Geometry: final body of the model. Coordinates: model frame, mm. Give positions to 0.01 mm unless a question says otherwise; leave off trailing zeros. Order: outer loops, then holes, each group sorted by start corner. A loop starts at its lowest first (then second) coordinate and runs counter-clockwise, first axis right, second up. Notation, with made-up numbers: (10, 19) -> (27, 19) arc R32 ccw to (27, 52) -> close; hole circle Ø6 at (63, 2). An arc over 180 degrees is marked (long way). Write item = value, one per line.
```python
from build123d import *

# Parameters (mm, degrees)
SKETCH1_R           = 1.8
BOSS_EXTRUDE1_DEPTH = 3


with BuildPart() as part:
    # Sketch1 → Boss-Extrude1 (new body)
    with BuildSketch(Plane(origin=(0, 0, 0), x_dir=(1, 0, 0), z_dir=(0, 1, 0))):
        with BuildLine():
            Line((11, 44), (11, 70))
            Line((11, 70), (0, 70))
            Line((0, 70), (0, 0))
            Line((0, 0), (11, 0))
            Line((11, 0), (11, 26))
            ThreePointArc((11, 26), (6.32455532, 35), (11, 44))
        make_face()
        with Locations((5.5, 65.5)):
            Circle(SKETCH1_R, mode=Mode.SUBTRACT)
        with Locations((5.5, 4.5)):
            Circle(SKETCH1_R, mode=Mode.SUBTRACT)
        with Locations((5.5, 19.5)):
            Circle(SKETCH1_R, mode=Mode.SUBTRACT)
        with Locations((5.5, 50.5)):
            Circle(SKETCH1_R, mode=Mode.SUBTRACT)
    extrude(amount=BOSS_EXTRUDE1_DEPTH)


solid = part.part
```
1) Section query A-A (x = 5.5). Output: boundary loops of the cut face in (y, z).
Check sheet entries:
outline = (0, -70) -> (3, -70) -> (3, -67.3) -> (0, -67.3) -> close; (0, -63.7) -> (3, -63.7) -> (3, -52.3) -> (0, -52.3) -> close; (0, -48.7) -> (3, -48.7) -> (3, -21.3) -> (0, -21.3) -> close; (0, -17.7) -> (3, -17.7) -> (3, -6.3) -> (0, -6.3) -> close; (0, -2.7) -> (3, -2.7) -> (3, 0) -> (0, 0) -> close
2) Mould query, pull axis Z, two halves, no side actions, for faces 1 (the face through (5.266, 1.479, -52.285)), 2 (the face through (11, 1, -57)), 3 (the face through (5, 1, 0)). Classes: +Z half, -Z half, draft (parallel to the pull), parting line (faces both ways), or undercut.
Check sheet entries:
face_1 = undercut
face_2 = draft
face_3 = +Z half
3) Section query B-B (z = -65.5). Output: boundary loops of the cut face in (x, y), plus the area to 3 significant figures.
Check sheet entries:
outline = (0, 0) -> (3.7, 0) -> (3.7, 3) -> (0, 3) -> close; (7.3, 0) -> (11, 0) -> (11, 3) -> (7.3, 3) -> close
area = 22.2 mm²
4) Section query C-C (y = 1). Output: boundary loops of the cut face in (x, z), plus the area to 3 significant figures.
Check sheet entries:
outline = (0, -70) -> (11, -70) -> (11, -44) arc R11 cw to (11, -26) -> (11, 0) -> (0, 0) -> close; hole circle Ø3.6 at (5.5, -65.5); hole circle Ø3.6 at (5.5, -50.5); hole circle Ø3.6 at (5.5, -19.5); hole circle Ø3.6 at (5.5, -4.5)
area = 670 mm²
5) Line query: line 1 (Z direction, x = 5.5, y = 1.95); line 2 (Z direction, x = 6, y = 0.7); line 3 (X direction, y = 2.05, z = -65.5). Output: solid intervals per line, ascending. Write a range as from..to.
Check sheet entries:
line_1 = -70..-67.3, -63.7..-52.3, -48.7..-21.3, -17.7..-6.3, -2.7..0
line_2 = -70..-67.23, -63.77..-52.23, -48.77..-21.23, -17.77..-6.23, -2.77..0
line_3 = 0..3.7, 7.3..11
